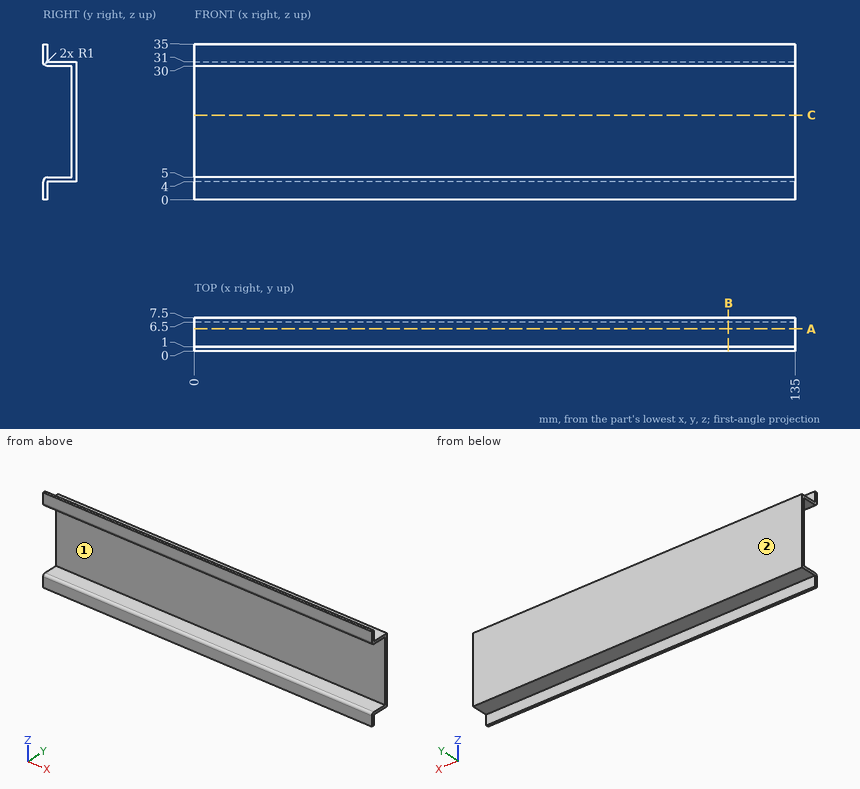
Could you check a few things on this drawing? It's one solid part, dimensions in mm from its lowest x, y, z. Round coordinates to 2 decimals unless told otherwise and drop trailing zeros. Order: outer loops, then holes, each group sorted by start corner. A loop starts at its lowest first (then second) coordinate and runs counter-clockwise, first axis right, second up. Notation, with made-up numbers: M -26,6.5 L -11,6.5 A14 ccw -11,10.5 Z; hole C 40,71 d7. An arc over 180 degrees is marked long. One line per question, with ' | ' between items. Start each with the question number.
(1) Suppose I cut it at A-A on y = 5. List the corners of the cut face in (x, z) for me, then the cut area to 3 significant figures.
(2) Thinking about a two-plate mould opening in Y: for the marked faces 1 and 2, which applies, +Y half, -Y half, draft (parallel to the pull), parting line (faces both ways), or undercut?
(3) Suppose I cut it at B-B on x = 120. List the corners of the cut face in (y, z) for me.
(4) Suppose I cut it at C-C on z = 19. List the corners of the cut face in (x, y) for me, then the cut area to 3 significant figures.
(5) For P1, Ø3, axis at x = 82.5, y = 3.5, coming from the -Z side; P2, Ø7.5, axis at x = 49.5, z = 17.5, coming from the -Y side; P3, Ø4.5, axis at x = 69, z = 33.5, coming from the +Y side, each with a flat end and sliding along its axis, tell me the tip position at first contact or that it passes through.
(6) Please list where these lines run through material, in increasing order: line 1 along Z through (x, y) = (67, 3.5); line 2 along Y through (x, z) = (58.5, 3); line 3 along Y through (x, z) = (82, 23.5).
Geometry results:
1) outline: M 0,4 L 135,4 L 135,5 L 0,5 Z; M 0,30 L 135,30 L 135,31 L 0,31 Z | area: 270 mm²
2) face 1: -Y half | face 2: +Y half
3) outline: M 0,0 L 1,0 L 1,4 L 7.5,4 L 7.5,31 L 1,31 L 1,35 L 0,35 L 0,31 A1 ccw 1,30 L 6.5,30 L 6.5,5 L 1,5 A1 ccw 0,4 Z
4) outline: M 0,6.5 L 135,6.5 L 135,7.5 L 0,7.5 Z | area: 135 mm²
5) P1: z = 4 | P2: y = 6.5 | P3: y = 1
6) line 1: 4 to 5, 30 to 31 | line 2: 0 to 1 | line 3: 6.5 to 7.5
